from build123d import *

# Parameters (mm, degrees)
F0_W          = 28.575
F0_H          = 28.575
F0_R          = 9.398
F1_DEPTH      = 2.3876
F2_DEPTH      = 13.3096
F2_DEPTH_BACK = 21.2344


with BuildPart() as f1:
    # F0 (on Front) → F1 (new body)
    with BuildSketch(Plane.XZ):
        Rectangle(F0_W, F0_H)
        Circle(F0_R, mode=Mode.SUBTRACT)
    extrude(amount=F1_DEPTH)

    # F0 (on Front) → F2 (join, two sides)
    with BuildSketch(Plane.XZ) as f2_sk:
        Circle(F0_R)
    extrude(amount=F2_DEPTH)
    extrude(f2_sk.sketch, amount=-F2_DEPTH_BACK)


solid = f1.part
Could you check a few things on this model? Use its own coordinates, in mm. A direction names the side the tool comes from. Give positions to 0.01 mm unless a question says otherwise; leave off trailing zeros. Write each loop counter-clockwise with the first axis right and the second up, starting at its lowest first coordinate (ties: lowest second). Pieces come first, ordered by that corner, then holes. Notation, with made-up numbers: (2.25, 52) -> (57.25, 52) arc R24 ccw to (57.25, 88) -> close; hole circle Ø1 at (71.25, 24.5). An arc over 180 degrees is marked (long way). Answer as a JSON object with one key per item and string values.
Q1. Which directions (+Z, -Z, +X, -X, +Y, -Y) give clear straight access to the entire face, cutting with the end or side of a thin tool? Please do faces 1 (the flat face through (0, -1, 14.288)), 2 (the cylindrical face through (-1.22, -7.77, 9.32)), 3 (the flat face through (0, 0, 10)).
Taken from the geometry:
{"face 1": "+Z, +X, -X, +Y, -Y", "face 2": "-Y", "face 3": "+Y"}
Q2. Suppose I cut it at D-D on z = 10. Write out the boundary of the cut face in (x, y).
Taken from the geometry:
{"outline": "(-14.29, -2.39) -> (14.29, -2.39) -> (14.29, 0) -> (-14.29, 0) -> close"}
Q3. Will these pins go through, and if not, where does the flat tip stop? pin 1 Ø6 at (x, z) = (-7.5, 10.5) entering from -Y; pin 2 Ø3 at (x, y) = (6, 15.5) entering from +Z.
Taken from the geometry:
{"pin 1": "stops at y = -2.39", "pin 2": "stops at z = 8.25"}
Q4. Suppose I cut it at B-B on z = 0. Write out the boundary of the cut face in (x, y), then the cut area to 3 significant figures.
Taken from the geometry:
{"outline": "(-14.29, -2.39) -> (-9.4, -2.39) -> (-9.4, -13.31) -> (9.4, -13.31) -> (9.4, -2.39) -> (14.29, -2.39) -> (14.29, 0) -> (9.4, 0) -> (9.4, 21.23) -> (-9.4, 21.23) -> (-9.4, 0) -> (-14.29, 0) -> close", "area": "673 mm²"}
Q5. Suppose I cut it at A-A on x = 0. Write out the boundary of the cut face in (y, z), then the cut area to 3 significant figures.
Taken from the geometry:
{"outline": "(-13.31, -9.4) -> (-2.39, -9.4) -> (-2.39, -14.29) -> (0, -14.29) -> (0, -9.4) -> (21.23, -9.4) -> (21.23, 9.4) -> (0, 9.4) -> (0, 14.29) -> (-2.39, 14.29) -> (-2.39, 9.4) -> (-13.31, 9.4) -> close", "area": "673 mm²"}
Q6. Suppose I cut it at C-C on y = 19.5. Write out the boundary of the cut face in (x, z), then the cut area to 3 significant figures.
Taken from the geometry:
{"outline": "circle Ø18.8 at (0, 0)", "area": "277 mm²"}
Q7. Please list where these lines run through material, in increasing order: L1, parallel to Y at x = 9.5, z = 8; L2, parallel to X at y = 7, z = -0.25; L3, parallel to X at y = -6, z = -5.75.
Taken from the geometry:
{"L1": "y = -2.39 to 0", "L2": "x = -9.39 to 9.39", "L3": "x = -7.43 to 7.43"}
